Check sheet for the modelled part. Datum: model origin and axes. Units: mm. A direction names the side the tool comes from. Give positions to 0.01 mm unless a question says otherwise; leave off trailing zeros. Loops run counter-clockwise (first coordinate to the right, second up) from the corner with the lowest first, then second, coordinate; pieces in that order, holes last. Notation, with made-up numbers: M 48,-0.75 L 104,-0.75 A22 cw 104,19.25 Z; hole C 69,-3 d10. An arc over 180 degrees is marked long. Use one line per item in the form item = value.
from build123d import *

# Parameters (mm, degrees)
SKETCH1_R                    = 14.2875
BOSS_EXTRUDE1_DEPTH          = 9.525
SKETCH2_W                    = 260.572878056
SKETCH2_H                    = 51.689000001
CUT_EXTRUDE1_DEPTH           = 10.525
SKETCH4_W                    = 213.36
SKETCH4_H                    = 68.767352002
CUT_EXTRUDE2_DEPTH           = 10.525
FILLET2_R                    = 25.4
SKETCH16_W                   = 9.525
SKETCH16_H                   = 4.28736328
CUT_EXTRUDE3_DEPTH           = 361.970011278
SKETCH17_W                   = 147.610011278
SKETCH17_H                   = 12.7
CUT_EXTRUDE4_DEPTH           = 10.525
TAP_DRILL_FOR_M6X0_75_TAP1_D = 5.25
F_6_4_6_4_DIAMETER_HOLE1_D   = 6.4
CUT_EXTRUDE5_DEPTH           = 10.525


with BuildPart() as part:
    # Sketch1 → Boss-Extrude1 (new body)
    with BuildSketch(Plane.XY):
        Polygon((-138.259383474, 48.991487021), (32.210627804, -121.478524257), (222.710627804, -121.478524257), (222.710627804, 149.508839023), (-138.259383474, 149.508839023), align=None)
        with Locations((180.538014078, 76.831975743)):
            Circle(SKETCH1_R, mode=Mode.SUBTRACT)
    extrude(amount=BOSS_EXTRUDE1_DEPTH)

    # Sketch2 → Cut-Extrude1 (cut, through all)
    with BuildSketch(Plane.XY.offset(9.525)):
        with Locations((111.474188776, -95.634024256)):
            Rectangle(SKETCH2_W, SKETCH2_H)
    extrude(amount=-CUT_EXTRUDE1_DEPTH, mode=Mode.SUBTRACT)

    # Sketch4 → Cut-Extrude2 (cut, through all)
    with BuildSketch(Plane.XY.offset(9.525)):
        with Locations((-31.579383474, 115.125163022)):
            Rectangle(SKETCH4_W, SKETCH4_H)
    extrude(amount=-CUT_EXTRUDE2_DEPTH, mode=Mode.SUBTRACT)

    # Fillet2
    fillet2_edges = [part.edges().sort_by_distance(p)[0] for p in [
        (-138.259383474, 80.741487021, 4.7625),
        (75.100616526, 80.741487021, 4.7625),
    ]]
    fillet(fillet2_edges, radius=FILLET2_R)

    # Sketch16 → Cut-Extrude3 (cut, through all)
    with BuildSketch(Plane(origin=(222.710627804, 0, 0), x_dir=(0, 0, -1), z_dir=(1, 0, 0))):
        with Locations((-4.7625, 147.365157383)):
            Rectangle(SKETCH16_W, SKETCH16_H)
    extrude(amount=-CUT_EXTRUDE3_DEPTH, mode=Mode.SUBTRACT)

    # Sketch17 → Cut-Extrude4 (cut, through all)
    with BuildSketch(Plane(origin=(0, 0, 0), x_dir=(-1, 0, 0), z_dir=(0, 0, -1))):
        with Locations((-148.905622165, 138.871475743)):
            Rectangle(SKETCH17_W, SKETCH17_H)
    extrude(amount=-CUT_EXTRUDE4_DEPTH, mode=Mode.SUBTRACT)

    # Tap Drill for M6x0.75 Tap1 (through all)
    with Locations(Plane.XY.offset(9.525)):
        with Locations((208.638014078, 104.931975743), (152.438014078, 104.931975743), (152.438014078, 48.731975743), (208.638014078, 48.731975743)):
            Hole(TAP_DRILL_FOR_M6X0_75_TAP1_D / 2)

    # Ø6.4 (6.4) Diameter Hole1 (through all)
    with Locations(Plane.XY.offset(9.525)):
        with Locations((196.040627804, -39.314524257), (60.150627804, -39.314524257), (-33.829372196, -39.314524257)):
            Hole(F_6_4_6_4_DIAMETER_HOLE1_D / 2)

    # Sketch22 → Cut-Extrude5 (cut, through all)
    with BuildSketch(Plane.XY.offset(9.525)):
        Polygon((-102.790372196, 145.085482826), (-102.790372196, -100.339530139), (-209.67575658, -95.573995907), (-209.67575658, 145.085482826), align=None)
    extrude(amount=-CUT_EXTRUDE5_DEPTH, mode=Mode.SUBTRACT)


solid = part.part
1) Scan lines: line 1 (X direction, y = 108.5, z = 7); line 2 (Y direction, x = 4.5, z = 1); line 3 (X direction, y = 78.5, z = 2.5). Record each from-to range of solid material in increasing order.
Evaluation:
line_1 = 75.1 to 222.71
line_2 = -69.79 to 80.74
line_3 = -102.79 to 166.35, 194.73 to 222.71
2) Section check D-D (x = 53.5). Record the cut outline in (y, z) (3 decimals), then the cut area to 3 significant figures.
Evaluation:
outline = M -69.79,0 L 81.027,0 L 81.027,9.525 L -69.79,9.525 Z
area = 1,440 mm^2
3) Set-up check for faces 5 (the face through (-61.39, -27.88, 4.7)), 6 (the face through (100, -69.79, 5)), 7 (the face through (-28, 80.741, 5)): record each of +Z, -Z, +X, -X, +Y, -Y from which the full face is reachable in a straight line by a thin tool's end or side.
Evaluation:
face_5 = +Z, -Z, -X, -Y
face_6 = +Z, -Z, +X, -Y
face_7 = +Z, -Z, -X, +Y
4) Section check C-C (y = 3). Record the cut outline in (x, z) (3 decimals), then the cut area to 3 significant figures.
Evaluation:
outline = M -92.268,0 L 222.711,0 L 222.711,9.525 L -92.268,9.525 Z
area = 3,000 mm^2
5) Release check for a two-part mould opening along X. For faces 1 (the face through (94, 32, 0)), 2 (the face through (-102.79, 48, 5)), 3 (the face through (-31.29, -41.26, 4.7)), 4 (the face through (170.01, 86.49, 4.7)) record: pulls with the +X half, pulls with the -X half, needs draft (parallel to the pull), parting line crosses it, or undercut.
Evaluation:
face_1 = needs draft
face_2 = pulls with the -X half
face_3 = undercut
face_4 = undercut
6) Section check A-A (x = 183). Record the cut outline in (y, z) (3 decimals), then the cut area to 3 significant figures.
Evaluation:
outline = M -69.79,0 L 62.758,0 L 62.758,9.525 L -69.79,9.525 Z; M 90.906,0 L 132.521,0 L 132.521,9.525 L 90.906,9.525 Z
area = 1,660 mm^2
7) Depth check by flat-ended pin: pin 1 Ø6 at (x, y) = (177.5, 94) entering from -Z; pin 2 Ø5 at (x, z) = (135.5, 2.5) entering from -Y; pin 3 Ø1 at (x, z) = (-68, 8) entering from -Y; pin 4 Ø3 at (y, z) = (116, 6) entering from -X. Enter the tip coordinate at first touch or a pass-through.
Evaluation:
pin_1 = 0
pin_2 = -69.79
pin_3 = -21.77
pin_4 = 75.1
8) Section check B-B (z = 4.5). State how many separate pieces and enclosed holes the cut face has, then the cut area to 3 significant figures.
Evaluation:
separate_pieces = 1
enclosed_holes = 8
area = 52,500 mm^2
